Check sheet for the modelled part. Datum: model origin and axes. Units: mm. A direction names the side the tool comes from. Give positions to 0.01 mm unless a question says otherwise; leave off trailing zeros. Loops run counter-clockwise (first coordinate to the right, second up) from the corner with the lowest first, then second, coordinate; pieces in that order, holes last. Notation, with made-up numbers: (41, 39.5) -> (80, 39.5) arc R23 ccw to (80, 72.5) -> close; hole circle Ø3 at (48, 86.25). An arc over 180 degrees is marked (long way). Write each question's results on one line, items separated by ' | '. Start each with the question number.
Item 1: Cross-section at C-C on x = 387. Enter the section's corners in (y, z), then the cut area to 3 significant figures.
Item 2: Gauge pin test, flat ends, axial feed: pin 1 Ø1.5 at (x, y) = (604.5, -109) entering from +Z; pin 2 Ø2 at (x, z) = (459, 1109.5) entering from -Y. Record the tip position at first contact, or that the pin passes through.
Item 3: Cross-section at A-A on y = -251. Enter the section's corners in (x, z), then the cut area to 3 significant figures.
Item 4: Access from +Z, -Z, +X, -X, +Y, -Y to the whole of each face (thin tool, end or side, straight path). Record for faces 5 (the face through (1061.829, -142, 622)), 6 (the face through (300, -141, -81.805)).
Item 5: Scan lines: line 1 along X through (y, z) = (-42, 969); line 2 along Z through (x, y) = (1, -132.5); line 3 along Y through (x, z) = (454.5, 1034.5). Record each from-to range of solid material in increasing order.
Item 6: Mould release check, pull along X, two halves, no side actions. Record for faces 1 (the face through (300, 0, 641)), 2 (the face through (300, -142, -79.265)), 3 (the face through (-442.706, -141, 621)), 4 (the face through (-440.166, -142, 622)): pulls with the +X half, pulls with the -X half, needs draft (parallel to the pull), parting line crosses it, or undercut.
Item 7: Cross-section at B-B on z = 1087.5. Enter the section's corners in (x, y), then the cut area to 3 significant figures.
from build123d import *

# Parameters (mm, degrees)
F0_W     = 1507.074781
F0_H     = 1424.91189
F1_DEPTH = 285.75
F2_T     = -2.54


with BuildPart() as f1:
    # F0 (on Front) → F1 (new body)
    with BuildSketch(Plane.XZ):
        with Locations((310.831803, 630.651133)):
            Rectangle(F0_W, F0_H)
    extrude(amount=F1_DEPTH)

    # F2
    f2_openings = [f1.faces().sort_by_distance(p)[0] for p in [
        (310.831804, -285.75, 630.651133),
        (310.831804, -142.875, 1343.107078),
    ]]
    offset(amount=F2_T, openings=f2_openings)


solid = f1.part
Answer sheet:
1) outline: (-285.75, -81.8) -> (0, -81.8) -> (0, 1343.11) -> (-2.54, 1343.11) -> (-2.54, -79.26) -> (-285.75, -79.26) -> close | area: 4,340 mm²
2) pin 1: stops at z = -79.26 | pin 2: stops at y = -2.54
3) outline: (-442.71, -81.8) -> (1064.37, -81.8) -> (1064.37, 1343.11) -> (1061.83, 1343.11) -> (1061.83, -79.26) -> (-440.17, -79.26) -> (-440.17, 1343.11) -> (-442.71, 1343.11) -> close | area: 11,100 mm²
4) face 5: +Z, -Y | face 6: -Z, +X, -X, +Y, -Y
5) line 1: x = -442.71 to -440.17, 1061.83 to 1064.37 | line 2: z = -81.8 to -79.26 | line 3: y = -2.54 to 0
6) face 1: needs draft | face 2: undercut | face 3: pulls with the -X half | face 4: undercut
7) outline: (-442.71, -285.75) -> (-440.17, -285.75) -> (-440.17, -2.54) -> (1061.83, -2.54) -> (1061.83, -285.75) -> (1064.37, -285.75) -> (1064.37, 0) -> (-442.71, 0) -> close | area: 5,270 mm²
